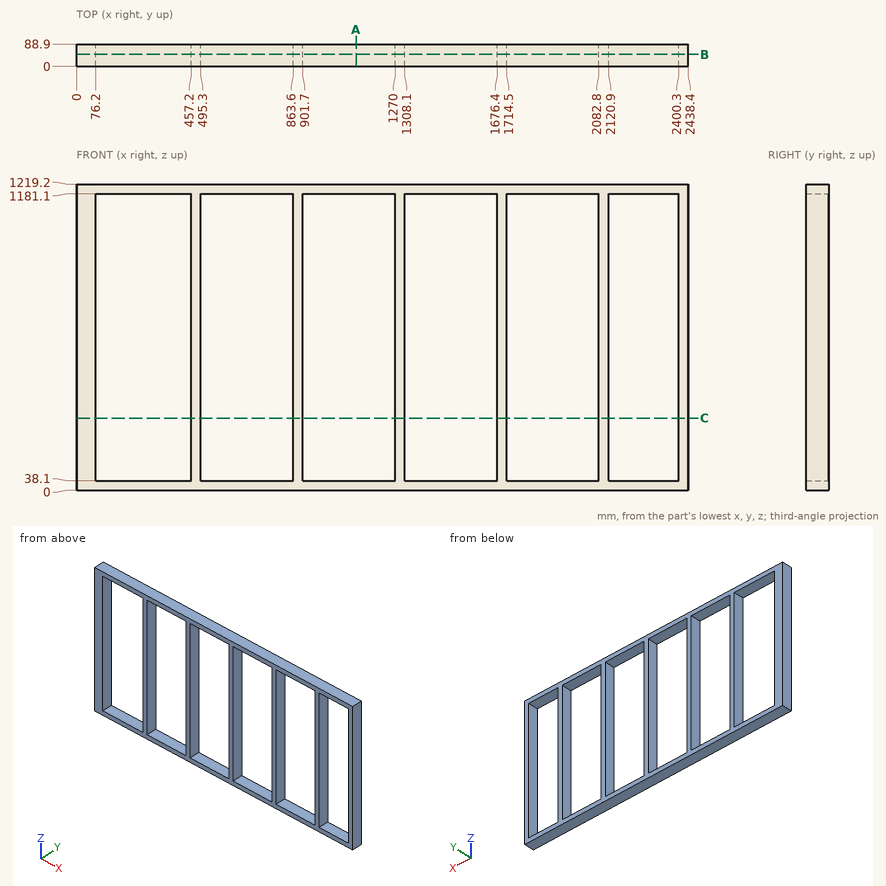
Here's the drawing with two shaded views (mm, measured from the low corner). I have some questions. Give positions to 0.01 mm unless a question says otherwise; leave off trailing zeros. Write each loop counter-clockwise with the first axis right and the second up, starting at its lowest first coordinate (ties: lowest second). Pieces come first, ordered by that corner, then holes. Notation, with made-up numbers: (-19.5, 12) -> (-13.5, 12) arc R7 cw to (-13.5, 23) -> close; hole circle Ø11 at (8, 47.25). An arc over 180 degrees is marked (long way). Use one line per item in the form item = value.
1) I'm going to push a flat-ended pin straight in: pin 1 (8 mm diameter, centred on x = 1978, y = 10, fed in from -Z). Where does the tip first touch, or does it pass through?
Verdict:
pin_1 = 0
2) Suppose I cut it at B-B (y = 48). Please give me the cut outline in (x, z), and give its area (3 significant figures).
Verdict:
outline = (0, 0) -> (2438.4, 0) -> (2438.4, 1219.2) -> (0, 1219.2) -> close; hole (76.2, 38.1) -> (457.2, 38.1) -> (457.2, 1181.1) -> (76.2, 1181.1) -> close; hole (495.3, 38.1) -> (863.6, 38.1) -> (863.6, 1181.1) -> (495.3, 1181.1) -> close; hole (901.7, 38.1) -> (1270, 38.1) -> (1270, 1181.1) -> (901.7, 1181.1) -> close; hole (1308.1, 38.1) -> (1676.4, 38.1) -> (1676.4, 1181.1) -> (1308.1, 1181.1) -> close; hole (1714.5, 38.1) -> (2082.8, 38.1) -> (2082.8, 1181.1) -> (1714.5, 1181.1) -> close; hole (2120.9, 38.1) -> (2400.3, 38.1) -> (2400.3, 1181.1) -> (2120.9, 1181.1) -> close
area = 534,000 mm2
3) Suppose I cut it at A-A (x = 1114.5). Please give me the cut outline in (y, z).
Verdict:
outline = (0, 0) -> (88.9, 0) -> (88.9, 38.1) -> (0, 38.1) -> close; (0, 1181.1) -> (88.9, 1181.1) -> (88.9, 1219.2) -> (0, 1219.2) -> close
4) If I drill on L1, parallel to Z at x = 1071.5, y = 75, over which ranges is the centre line in solid material (lowest first)? Write a range as [from, to].
Verdict:
L1 = [0, 38.1], [1181.1, 1219.2]
5) Suppose I cut it at C-C (z = 287). Please give me the cut outline in (x, y).
Verdict:
outline = (0, 0) -> (76.2, 0) -> (76.2, 88.9) -> (0, 88.9) -> close; (457.2, 0) -> (495.3, 0) -> (495.3, 88.9) -> (457.2, 88.9) -> close; (863.6, 0) -> (901.7, 0) -> (901.7, 88.9) -> (863.6, 88.9) -> close; (1270, 0) -> (1308.1, 0) -> (1308.1, 88.9) -> (1270, 88.9) -> close; (1676.4, 0) -> (1714.5, 0) -> (1714.5, 88.9) -> (1676.4, 88.9) -> close; (2082.8, 0) -> (2120.9, 0) -> (2120.9, 88.9) -> (2082.8, 88.9) -> close; (2400.3, 0) -> (2438.4, 0) -> (2438.4, 88.9) -> (2400.3, 88.9) -> close
